Geometry: final body of the model. Coordinates: model frame, mm. A direction names the side the tool comes from. Round coordinates to 2 decimals unless told otherwise and drop trailing zeros. Loops run counter-clockwise (first coordinate to the right, second up) from the corner with the lowest first, then second, coordinate; pieces in that order, holes last. Notation, with made-up numbers: M 75.5,89 L 109.5,89 A23 cw 109.5,124 Z; hole C 35.5,70.5 d6. An arc over 180 degrees is marked long. Answer as a JSON object with one key per item and string values.
Autodesk Inventor part; units mm, degrees
ref_plane "YZ Plane" through (0, 0, 0) normal (1, 0, 0) x (0, 1, 0)
ref_plane "XZ Plane" through (0, 0, 0) normal (0, 1, 0) x (-1, 0, 0)
ref_plane "XY Plane" through (0, 0, 0) normal (0, 0, 1) x (1, 0, 0)
sketch "Sketch5" plane through (0, 0, 0) normal (0, 0, 1) x (1, 0, 0)
  line L0 (52.8, -15.6) -> (52.8, -10.6)
  line L1 (52.8, -10.6) -> (49.8, -10.6)
  line L2 (49.8, -10.6) -> (49.8, -12.6)
  line L3 (44, -12.6) -> (44, -3)
  line L4 (49.8, -3) -> (49.8, -5)
  line L5 (49.8, -5) -> (52.8, -5)
  line L6 (52.8, -5) -> (52.8, 0)
  line L7 (52.8, 0) -> (7.8, 0)
  line L8 (44, -3) -> (49.8, -3)
  line L9 (44, -12.6) -> (49.8, -12.6)
  line L10 (52.8, -15.6) -> (7.8, -15.6)
  line L11 (7.8, -15.6) -> (0, -15.6)
  line L12 (0, -15.6) -> (0, 0)
  line L13 (0, 0) -> (7.8, 0)
  point P0 (7.8, 0)
  dimension "d41" = 5.8
  dimension "d48" = 44
  dimension "d50" = 3
  dimension "d63" = 45
  dimension "d71" = 0
  dimension "d87" = 5.6
  dimension "d88" = 9.6
  dimension "d97" = 15.6
extrude "Extrusion2" add sketch "Sketch5" along normal blind 12
sketch "Sketch8" plane through (0, 0, 0) normal (0, 0, -1) x (-1, 0, 0)
  line L0 (-8.1687, 0) -> (-8.8633, -3.9392)
  line L1 (-7.8, 0) -> (-1.143, 0) construction
  line L2 (0, -5.5021) -> (-8.8633, -3.9392)
  line L3 (-7.8, 0) -> (-8.1687, 0)
  line L4 (0, 0) -> (0, -15.6)
  line L5 (-52.8, 0) -> (0, 0)
  line L6 (-7.8, 0) -> (0, 0)
  line L7 (0, 0) -> (0, -5.5021)
  dimension "d80" = 100
  dimension "d95" = 4
  dimension "d96" = 9
extrude "Extrusion5" cut sketch "Sketch8" against normal through all
fillet "Fillet2" radius 23 1 edges at (0, -15.6, 6)
equation "\"l1\" = 8"
properties part number "Finray_test_8_Kerbe_10deg"
1) Section query B-B (y = -9.5). Return the cut outline in (x, z), and give its area (3 significant figures).
Results:
{"outline": "M 3.44,0 L 44,0 L 44,12 L 3.44,12 Z", "area": "487 mm2"}
2) Ray query, line 1 (Y direction, x = 46, z = 8); line 2 (Y direction, x = 50, z = 0.5); line 3 (X direction, y = -11, z = 9.5). Return the intervals inside material, ascending.
Results:
{"line 1": "-15.6 to -12.6, -3 to 0", "line 2": "-15.6 to -10.6, -5 to 0", "line 3": "5.24 to 44, 49.8 to 52.8"}
3) Section query A-A (z = 2.5). Return the cut outline in (x, y).
Results:
{"outline": "M 0,-5.5 A23 ccw 19.04,-15.6 L 52.8,-15.6 L 52.8,-10.6 L 49.8,-10.6 L 49.8,-12.6 L 44,-12.6 L 44,-3 L 49.8,-3 L 49.8,-5 L 52.8,-5 L 52.8,0 L 8.17,0 L 8.86,-3.94 Z"}
4) Pin query (flat end, axial travel): P1, Ø0.6, axis at y = -11.5, z = 4, coming from the -X side. Return the tip coordinate at first contact, or that it passes through.
Results:
{"P1": "x = 5.51"}
5) Pull-direction query (X, two-part tool) for faces 1 (the flat face through (52.8, -13, 6)), 2 (the flat face through (49.8, -12, 6)), 3 (the flat face through (51, -5, 6)); classes: +X half, -X half, draft (parallel to the pull), parting line (faces both ways), or undercut.
Results:
{"face 1": "+X half", "face 2": "undercut", "face 3": "draft"}
6) Reachability of faces 4 (the flat face through (8.51, -1.94, 5.92)), 5 (the flat face through (51, -10.6, 6)), 6 (the flat face through (47, -12.6, 6)), 7 (the flat face through (26, -8, 12)) from +Z, -Z, +X, -X, +Y, -Y: full face, straight path, thin tool, end or side. Return the list, or none.
Results:
{"face 4": "+Z, -Z, -X", "face 5": "+Z, -Z, +X", "face 6": "+Z, -Z", "face 7": "+Z, +X, -X, +Y, -Y"}
7) Section query C-C (x = 4). Return the cut outline in (y, z), and give its area (3 significant figures).
Results:
{"outline": "M -10,0 L -4.8,0 L -4.8,12 L -10,12 Z", "area": "62.4 mm2"}
